Check sheet for the modelled part. Datum: model origin and axes. Units: mm. A direction names the side the tool comes from. Coordinates: 2 decimals unless noted, no trailing zeros. Loops run counter-clockwise (first coordinate to the right, second up) from the corner with the lowest first, then second, coordinate; pieces in that order, holes last. Notation, with made-up numbers: (-30.5, -2) - (25.5, -2) arc R15 cw to (25.5, 27) - close; hole circle Ø9 at (50, 40.25). An arc over 180 degrees is marked (long way). Write each question's results on one line, items separated by ' | '. Start each with the question number.
1. Cross-section at C-C (z = -135.5). Record the cut outline in (x, y).
2. Tool access check on faces 1 (the face through (-273, -13, -381)), 2 (the face through (-241.3, -13, -444)), 3 (the face through (-273, -13, -508)), 4 (the face through (-72.43, 19.32, -812.62)), 5 (the face through (-279, 19, 0)). Record the directions out of +Z, -Z, +X, -X, +Y, -Y that give a thin tool (end or side, any length) a straight path to the whole face; none if there is none.
3. Cross-section at A-A (y = 19.5). Record the cut outline in (x, z).
4. Gauge pin test, flat ends, axial feed: P1, Ø5, axis at x = -116, y = 18, coming from the -Z side; P2, Ø1, axis at x = -160.5, y = 7.5, coming from the +Z side; P3, Ø12, axis at x = -139.5, y = 28, coming from the -Z side. Record the tip position at first contact, or that the pin passes through.
5. Cross-section at B-B (x = -197). Record the cut outline in (y, z).
6. Thickness scan on line 1 (Y direction, x = -181.5, z = -544); line 2 (Z direction, x = -248, y = 6.5); line 3 (Z direction, x = -242, y = -1). Record the ranges inside material, lowest first. Write a range as [from, to].
Autodesk Inventor part; units mm, degrees
ref_plane "YZ Plane" through (0, 0, 0) normal (1, 0, 0) x (0, 1, 0)
ref_plane "XZ Plane" through (0, 0, 0) normal (0, 1, 0) x (-1, 0, 0)
ref_plane "XY Plane" through (0, 0, 0) normal (0, 0, 1) x (1, 0, 0)
sketch "Sketch1" plane through (0, 0, 0) normal (0, 1, 0) x (-1, 0, 0)
  line L0 (0, 0) -> (304.8, 0)
  line L1 (304.8, 0) -> (304.8, -889)
  line L2 (304.8, -889) -> (0, -889)
  line L3 (0, -889) -> (0, 0)
  dimension "d0" = 889
  dimension "d1" = 304.8
extrude "Extrusion1" add sketch "Sketch1" along normal blind 38.1
fillet "Fillet1" radius 254 1 edges at (0, 19.05, 0)
fillet "Fillet2" radius 254 1 edges at (0, 19.05, -889)
sketch "Sketch2" plane through (0, 0, 0) normal (0, -1, 0) x (1, 0, 0)
  line L0 (-254, -889) -> (-304.8, -889)
  line L1 (-304.8, -889) -> (-304.8, 0)
  line L2 (-304.8, -889) -> (-304.8, 0)
  line L3 (-304.8, 0) -> (-304.8, -381)
  line L4 (-304.8, -381) -> (-241.3, -381)
  line L5 (-241.3, -381) -> (-241.3, -508)
  line L6 (-241.3, -508) -> (-304.8, -508)
  line L7 (-304.8, -889) -> (-304.8, -508)
  line L8 (-304.8, -508) -> (-241.3, -508)
  line L9 (-241.3, -508) -> (-241.3, -381)
  line L10 (-241.3, -381) -> (-304.8, -381)
  point P0 (0, 0)
  dimension "d6" = 381
  dimension "d7" = 63.5
  dimension "d8" = 127
  dimension "d9" = 381
  dimension "d10" = 127
extrude "Extrusion2" add sketch "Sketch2" along normal blind 25.4
properties part number "Shelf-ver2-1111-2021" material "Aluminum 6061"
Established:
1) outline: (-304.8, 0) - (-29.34, 0) - (-29.34, 38.1) - (-304.8, 38.1) - close
2) face 1: +Z, +X, -X, -Y | face 2: +Z, -Z, +X, -Y | face 3: -Z, +X, -X, -Y | face 4: -Z, +X, +Y, -Y | face 5: +Z, +X, -X, +Y, -Y
3) outline: (-304.8, -889) - (-254, -889) arc R254 ccw to (0, -635) - (0, -254) arc R254 ccw to (-254, 0) - (-304.8, 0) - close
4) P1: z = -849.84 | P2: z = -17.64 | P3: z = -864.66
5) outline: (0, -882.52) - (38.1, -882.52) - (38.1, -6.48) - (0, -6.48) - close
6) line 1: [0, 38.1] | line 2: [-888.93, -0.07] | line 3: [-508, -381]
